Geometry check sheet. Reference: drawing and pictorial views, mm from the part's lowest x, y, z. A direction names the side the tool comes from. Round coordinates to 2 decimals unless told otherwise and drop trailing zeros. Order: outer loops, then holes, each group sorted by start corner. A loop starts at its lowest first (then second) coordinate and runs counter-clockwise, first axis right, second up.
(1) Cross-section at C-C on z = 9.5. Enter the section's corners in (x, y) (3 decimals).
(2) Set-up check for the marked faces 5, 6 and 7: record each of +Z, -Z, +X, -X, +Y, -Y from which the full face is reachable in a straight line by a thin tool's end or side.
(3) Cross-section at A-A on y = 2. Enter the section's corners in (x, z).
(4) Gauge pin test, flat ends, axial feed: P1, Ø3, axis at x = 5, y = 18.5, coming from the +Z side; P2, Ø5, axis at x = 25.5, y = 26.5, coming from the +Z side; P3, Ø2, axis at x = 7.5, z = 7.5, coming from the -Y side. Record the tip position at first contact, or that the pin passes through.
(5) Cross-section at B-B on x = 12.5. Enter the section's corners in (y, z).
(6) Thickness scan on L1, parallel to Y at x = 16.5, z = 10.75; L2, parallel to Y at x = 21.5, z = 5. Record the ranges inside material, lowest first.
(7) Draft check along Y on the marked faces 1, 2, 3 and 4. Enter one of: pulls with the +Y half, pulls with the -Y half, needs draft (parallel to the pull), parting line crosses it, or undercut.
(8) Cross-section at D-D on x = 6.5. Enter the section's corners in (y, z).
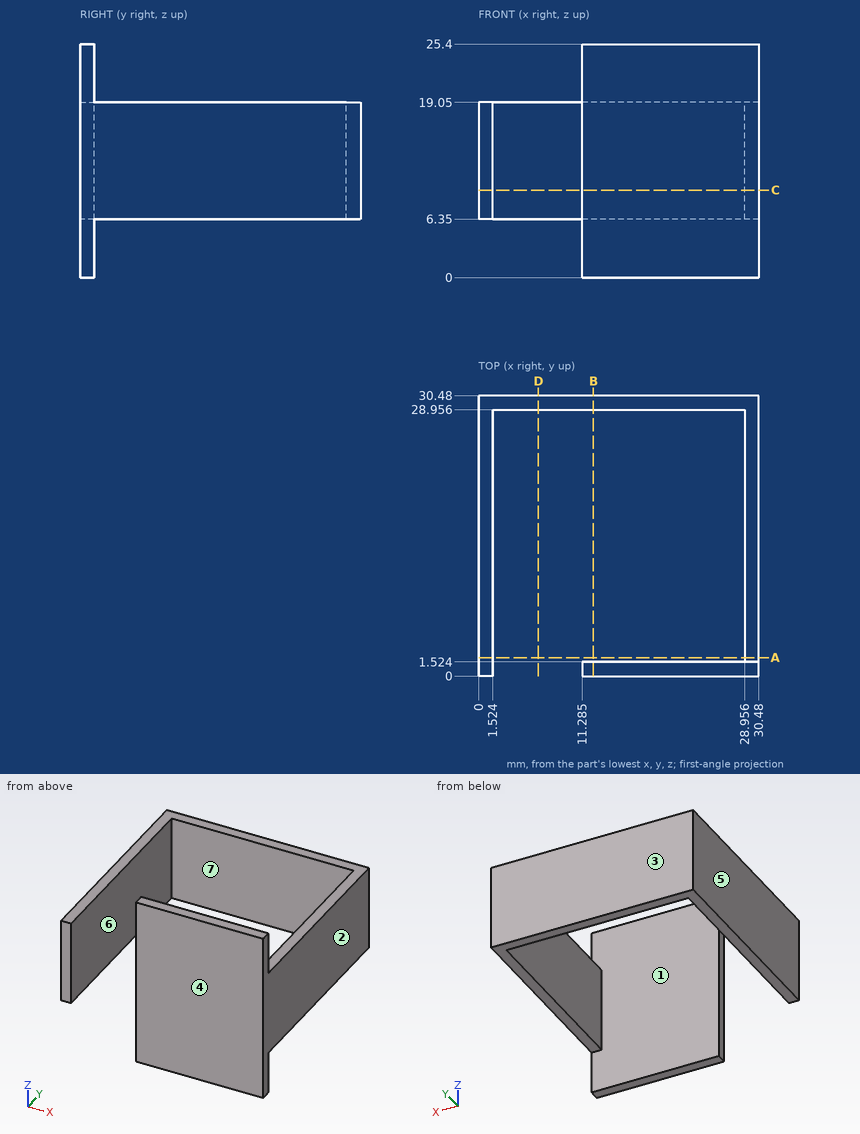
Found:
1. outline: (0, 0) - (1.524, 0) - (1.524, 28.956) - (28.956, 28.956) - (28.956, 1.524) - (11.285, 1.524) - (11.285, 0) - (30.48, 0) - (30.48, 30.48) - (0, 30.48) - close
2. face 5: +Z, -Z, -X, +Y, -Y
2. face 6: +Z, -Z, -Y
2. face 7: +Z, -Z
3. outline: (0, 6.35) - (1.52, 6.35) - (1.52, 19.05) - (0, 19.05) - close; (28.96, 6.35) - (30.48, 6.35) - (30.48, 19.05) - (28.96, 19.05) - close
4. P1: passes through
4. P2: stops at z = 19.05
4. P3: stops at y = 28.96
5. outline: (0, 0) - (1.52, 0) - (1.52, 25.4) - (0, 25.4) - close; (28.96, 6.35) - (30.48, 6.35) - (30.48, 19.05) - (28.96, 19.05) - close
6. L1: y = 0 to 1.52, 28.96 to 30.48
6. L2: y = 0 to 1.52
7. face 1: undercut
7. face 2: needs draft
7. face 3: pulls with the +Y half
7. face 4: pulls with the -Y half
8. outline: (28.96, 6.35) - (30.48, 6.35) - (30.48, 19.05) - (28.96, 19.05) - close
